from build123d import *


with BuildPart() as f1:
    # F0 (on Front) → F1 (revolve)
    with BuildSketch(Plane.XZ):
        with BuildLine():
            Line((0, 4.193819), (0, 0))
            Line((0, 0), (30.459946, 0))
            Line((30.459946, 0), (49.550053, -11.931316))
            Line((49.550053, -11.931316), (57.517636, -11.931316))
            ThreePointArc((57.517636, -11.931316), (62.007764, -10.071444), (63.867636, -5.581316))
            Line((63.867636, -5.581316), (63.867636, 73.131949))
            Line((63.867636, 73.131949), (63.867636, 112.469681))
            Line((63.867636, 112.469681), (39.425094, 135.337606))
            Line((39.425094, 135.337606), (39.425094, 153.195813))
            Line((39.425094, 153.195813), (33.017382, 153.195813))
            Line((33.017382, 153.195813), (33.017382, 135.337606))
            Line((33.017382, 135.337606), (57.459924, 112.469681))
            Line((57.459924, 112.469681), (57.459924, -6.803995))
            Line((57.459924, -6.803995), (50.88336, -6.803995))
            Line((50.88336, -6.803995), (39.425094, 0))
            Line((39.425094, 0), (34.942501, 4.193819))
            Line((34.942501, 4.193819), (6.416916, 4.193819))
            Line((6.416916, 4.193819), (0, 4.193819))
        make_face()
    revolve(axis=Axis((0, 0, 36.565974), (0, 0, 1)))


solid = f1.part
Here's how the part is built. I have some questions about the finished solid (model axes, mm). A direction names the side the tool comes from. Coordinates: 2 decimals unless noted, no trailing zeros. Write each loop counter-clockwise with the first axis right and the second up, starting at its lowest first coordinate (ties: lowest second). Pieces come first, ordered by that corner, then holes. Notation, with made-up numbers: (-16.75, -4.5) - (32.25, -4.5) arc R18 cw to (32.25, 25.5) - close; hole circle Ø2 at (29.25, 50). An arc over 180 degrees is marked (long way). Use one line per item in the form item = value.
1) Suppose I cut it at A-A, the plane x = 0. Write out the boundary of the cut face in (y, z), plus the area to 3 significant figures.
Solved:
outline = (-63.87, -5.58) arc R6.35 ccw to (-57.52, -11.93) - (-49.55, -11.93) - (-30.46, 0) - (30.46, 0) - (49.55, -11.93) - (57.52, -11.93) arc R6.35 ccw to (63.87, -5.58) - (63.87, 112.47) - (39.43, 135.34) - (39.43, 153.2) - (33.02, 153.2) - (33.02, 135.34) - (57.46, 112.47) - (57.46, -6.8) - (50.88, -6.8) - (39.43, 0) - (34.94, 4.19) - (-34.94, 4.19) - (-39.43, 0) - (-50.88, -6.8) - (-57.46, -6.8) - (-57.46, 112.47) - (-33.02, 135.34) - (-33.02, 153.2) - (-39.43, 153.2) - (-39.43, 135.34) - (-63.87, 112.47) - close
area = 2,660 mm2
2) I'm going to push flat-ended pins straight in: P1, Ø18.5, axis at x = -5.5, y = -12.5, coming from the -Z side; P2, Ø1.5, axis at y = 31, z = 36.5, coming from the +X side; P3, Ø12, axis at x = 12, z = 56, coming from the -Y side. Where does each tip first touch, or does it pass through?
Solved:
P1 = 0
P2 = 56.25
P3 = -63.59
3) Thinking about a two-plate mould opening in Z: for faces 4 (the conical face through (-27.902, -21.394, 3.99)), 5 (the cylindrical face through (-8.547, -38.488, 144.392)), 6 (the flat face through (-17, 47, -11.931)), which applies, released by +Z, released by -Z, zero draft, split by the parting line, or undercut?
Solved:
face_4 = undercut
face_5 = zero draft
face_6 = released by -Z
4) I need wall thicknesses on line 1 (Y direction, x = 0, z = 149); line 2 (Y direction, x = 0, z = 63); line 3 (Z direction, x = -41.5, y = -12). Which ranges of each line are inside material? Lowest first, please.
Solved:
line_1 = -39.43 to -33.02, 33.02 to 39.43
line_2 = -63.87 to -57.46, 57.46 to 63.87
line_3 = -7.96 to -2.24, 125.81 to 131.81
5) On a 3-axis mill with a long thin cutter (end or side, diameter ignored), from which of +Z, -Z, +X, -X, +Y, -Y can I reach the whole of each face in a straight line? I mean faces 1 (the cylindrical face through (-26.2, -20.09, 144.14)), 2 (the flat face through (-5, -51, -6.804)), 3 (the flat face through (0, 0, 0)). Say none if no direction works.
Solved:
face_1 = +Z
face_2 = none
face_3 = -Z
6) Suppose I cut it at C-C, the plane z = 50. Write out the boundary of the cut face in (x, y), plus the area to 3 significant figures.
Solved:
outline = circle Ø127.74 at (0, 0); hole circle Ø114.92 at (0, 0)
area = 2,440 mm2
